Check sheet for the modelled part. Datum: model origin and axes. Units: mm. Face numbers are marked on the shaded views. A direction names the side the tool comes from. Give positions to 0.01 mm unless a question says otherwise; leave off trailing zeros. Order: outer loops, then holes, each group sorted by start corner. A loop starts at its lowest first (then second) coordinate and runs counter-clockwise, first axis right, second up.
Item 1: Access from +Z, -Z, +X, -X, +Y, -Y to the whole of each face (thin tool, end or side, straight path). Record for the marked faces 4 and 5.
Item 2: Sectioned sample at A-A on y = 0. Record the boundary of the cut face in (x, z).
Item 3: Sectioned sample at D-D on x = -12. Record the boundary of the cut face in (y, z).
Item 4: Material ranges on line 1 along Y through (x, z) = (-4, -1.5); line 2 along Z through (x, y) = (13, -5.5); line 3 along X through (y, z) = (-3, -11), recorded low to high.
Item 5: Release check for a two-part mould opening along X. For the marked faces 1, 2 and 3 record: released by +X, released by -X, zero draft, split by the parting line, or undercut.
Item 6: Gauge pin test, flat ends, axial feed: P1, Ø12, axis at x = -11, z = 0.5, coming from the +Y side; P2, Ø5, axis at x = -5.5, z = -9, coming from the +Y side; P3, Ø6.5, axis at x = 0, y = 0, coming from the -Z side; P4, Ø8, axis at x = 10, z = -23.5, coming from the -Y side. Record the tip position at first contact, or that the pin passes through.
Item 7: Sectioned sample at B-B on x = 0. Record the boundary of the cut face in (y, z).
Item 8: Sectioned sample at C-C on z = -24.5. Record the boundary of the cut face in (x, y).
from build123d import *

# Parameters (mm, degrees)
SKETCH1_R                  = 5.5
SKETCH1_R_2                = 2.4
BOSS_EXTRUDE1_DEPTH        = 4
BOSS_EXTRUDE2_START        = 27
SKETCH2_R                  = 11
SKETCH2_R_2                = 5.5
BOSS_EXTRUDE2_DEPTH        = 27
M8X1_25_TAPPED_HOLE1_D     = 6.8
M8X1_25_TAPPED_HOLE1_DEPTH = 8
M8X1_25_TAPPED_HOLE1_TIP   = 2.042926105


with BuildPart() as part:
    # Sketch1 → Boss-Extrude1 (new, symmetric)
    with BuildSketch(Plane.XY):
        with BuildLine():
            Line((-15, 13.228756555), (-15, -13.228756555))
            ThreePointArc((-15, -13.228756555), (0, -20), (15, -13.228756555))
            Line((15, -13.228756555), (15, 13.228756555))
            ThreePointArc((15, 13.228756555), (0, 20), (-15, 13.228756555))
        make_face()
        Circle(SKETCH1_R, mode=Mode.SUBTRACT)
        with Locations((-11.313708499, 11.313708499)):
            Circle(SKETCH1_R_2, mode=Mode.SUBTRACT)
        with Locations((0, 16)):
            Circle(SKETCH1_R_2, mode=Mode.SUBTRACT)
        with Locations(Location((11.313708499, 11.313708499, 0), (0, 0, 180))):
            Circle(SKETCH1_R_2, mode=Mode.SUBTRACT)
        with Locations((11.313708499, -11.313708499)):
            Circle(SKETCH1_R_2, mode=Mode.SUBTRACT)
        with Locations(Location((0, -16, 0), (0, 0, 180))):
            Circle(SKETCH1_R_2, mode=Mode.SUBTRACT)
        with Locations(Location((-11.313708499, -11.313708499, 0), (0, 0, 180))):
            Circle(SKETCH1_R_2, mode=Mode.SUBTRACT)
    extrude(amount=BOSS_EXTRUDE1_DEPTH, both=True)

    # Sketch2 → Boss-Extrude2 (add)
    with BuildSketch(Plane(origin=(0, 0, -4), x_dir=(-1, 0, 0), z_dir=(0, 0, -1)).offset(BOSS_EXTRUDE2_START)):
        with Locations(Location((0, 0, 0), (0, 0, 180))):
            Circle(SKETCH2_R)
        with Locations(Location((0, 0, 0), (0, 0, 180))):
            Circle(SKETCH2_R_2, mode=Mode.SUBTRACT)
    extrude(amount=-BOSS_EXTRUDE2_DEPTH)

    # M8x1.25 Tapped Hole1
    with Locations(Plane(origin=(-7.653668647, 18.47759065, 0), x_dir=(0.923879532511, 0.382683432365, 0), z_dir=(-0.382683432365, 0.923879532511, 0))):
        with Locations((0, 0)):
            Hole(M8X1_25_TAPPED_HOLE1_D / 2, depth=M8X1_25_TAPPED_HOLE1_DEPTH)
            with Locations((0, 0, -(M8X1_25_TAPPED_HOLE1_DEPTH + M8X1_25_TAPPED_HOLE1_TIP / 2))):  # 118° drill point
                Cone(0, M8X1_25_TAPPED_HOLE1_D / 2, M8X1_25_TAPPED_HOLE1_TIP, mode=Mode.SUBTRACT)


solid = part.part
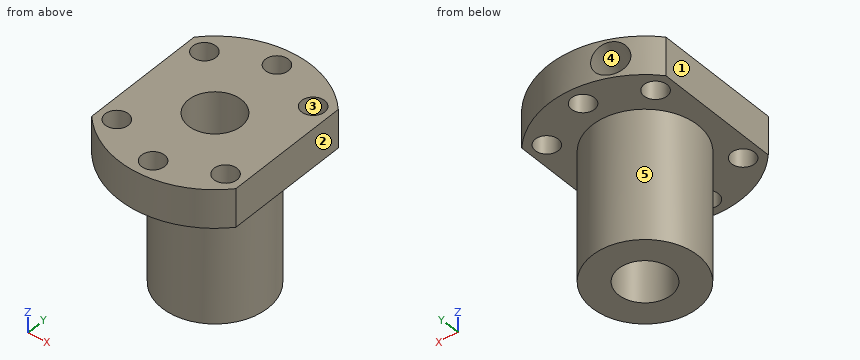
Report:
1. face 4: none
1. face 5: -Z
2. outline: (-15, -4) - (-11, -4) - (-11, -31) - (-5.5, -31) - (-5.5, 4) - (-15, 4) - close; (5.5, -31) - (11, -31) - (11, -4) - (15, -4) - (15, 4) - (5.5, 4) - close
3. outline: (-16, -4) - (-13.61, -4) - (-13.61, 4) - (-16, 4) - close; (-9.01, -4) - (9.01, -4) - (9.01, 4) - (-9.01, 4) - close; (13.61, -4) - (16, -4) - (16, 4) - (13.61, 4) - close
4. line 1: y = -19.6 to -3.77, 3.77 to 10.1, 17.63 to 19.6
4. line 2: z = -4 to 4
4. line 3: x = -10.58 to -4.61, 4.61 to 10.58
5. face 1: released by -X
5. face 2: released by +X
5. face 3: undercut
6. P1: stops at y = 19.29
6. P2: stops at y = 10.58
6. P3: passes through
6. P4: stops at y = -9.22
7. outline: (-20, -4) - (-18.4, -4) - (-18.4, 4) - (-20, 4) - close; (-13.6, -4) - (-11, -4) - (-11, -31) - (-5.5, -31) - (-5.5, 4) - (-13.6, 4) - close; (5.5, -31) - (11, -31) - (11, -4) - (13.6, -4) - (13.6, 4) - (5.5, 4) - close; (18.4, -4) - (20, -4) - (20, 4) - (18.4, 4) - close
8. outline: circle Ø22 at (0, 0); hole circle Ø11 at (0, 0)
